Autodesk Inventor part; units mm, degrees
ref_plane "YZ Plane" through (0, 0, 0) normal (1, 0, 0) x (0, 1, 0)
ref_plane "XZ Plane" through (0, 0, 0) normal (0, 1, 0) x (-1, 0, 0)
ref_plane "XY Plane" through (0, 0, 0) normal (0, 0, 1) x (1, 0, 0)
sketch "Sketch1" plane through (0, 0, 0) normal (0, 1, 0) x (-1, 0, 0)
  circle A0 centre (0, 0) radius 69.85
  dimension "d0" = 139.7
extrude "Extrusion1" add sketch "Sketch1" along normal blind 29.21
sketch "Sketch3" plane through (0, 29.21, 0) normal (0, 1, 0) x (1, 0, 0)
  circle A0 centre (0, 0) radius 67.31
  dimension "d5" = 134.62
extrude "Extrusion2" cut sketch "Sketch3" against normal blind 26.67
sketch "Sketch6" plane through (0, 0, 0) normal (1, 0, 0) x (0, 1, 0)
  line L0 (29.21, 67.31) -> (2.54, 67.31)
  line L1 (29.21, 67.31) -> (27.686, 67.31)
  line L2 (27.686, 67.31) -> (27.686, 65.024)
  line L3 (27.686, 65.024) -> (29.21, 65.024)
  line L4 (29.21, 65.024) -> (29.21, 67.31)
  line L5 (-5.842, 0) -> (35.052, 0)
  line L6 (29.21, -69.85) -> (29.21, 69.85)
  point P0 (0, 0)
  dimension "d21" = 1.524
  dimension "d22" = 2.286
  dimension "d36" = 0
revolve "Revolution1" add sketch "Sketch6" angle 30 about axis through (0, -10, 0) along (0, 1, 0)
fillet "Fillet2" radius 0.762 2 edges at (16.8294, 27.686, 62.8084) (16.8294, 29.21, 62.8084)
fillet "Fillet3" radius 0.762 3 edges at (32.6235, 27.909, 56.5056) (33.2739, 29.21, 57.632) (33.2739, 27.686, 57.632)
pattern_circular "Circular Pattern1" count 3 over 360 about axis through (0, 0, 0) along (0, 1, 0) of "Revolution1", "Fillet2", "Fillet3"
sketch "Sketch9" plane through (0, 0, 0) normal (1, 0, 0) x (0, 1, 0)
  circle A0 centre (6.8717, 0) radius 3.175 construction
  line L0 (6.8717, 0) -> (6.8717, -12.7) construction
  line L1 (6.8717, 0) -> (6.8717, 12.7) construction
  line L2 (6.8717, -12.7) -> (6.8717, -12.7)
  line L3 (3.6967, -9.525) -> (3.6967, 9.525)
  line L4 (6.8717, 12.7) -> (6.8717, 12.7)
  line L5 (10.0467, 9.525) -> (10.0467, -9.525)
  arc A1 (6.8717, -12.7) -> (10.0467, -9.525) centre (6.8717, -9.525) ccw
  arc A2 (3.6967, -9.525) -> (6.8717, -12.7) centre (6.8717, -9.525) ccw
  arc A3 (6.8717, 12.7) -> (3.6967, 9.525) centre (6.8717, 9.525) ccw
  arc A4 (10.0467, 9.525) -> (6.8717, 12.7) centre (6.8717, 9.525) ccw
  point P0 (0, 0)
  dimension "d37" = 6.35
  dimension "d48" = 12.7
  dimension "d49" = 12.7
  dimension "d50" = 3.175
extrude "Extrusion9" cut sketch "Sketch9" along normal through all
sketch "Sketch20" plane through (0, 2.54, 0) normal (0, 1, 0) x (1, 0, 0)
  circle A0 centre (0, 0) radius 3.4925
  circle A1 centre (13.4366, 0) radius 24.638
  line L0 (38.0746, 0) -> (30.4546, 0) construction
  line L1 (30.4546, 0) -> (30.4546, -17.8162)
  line L2 (30.4546, 0) -> (30.4546, 17.8162)
  dimension "d70" = 6.985
  dimension "d71" = 49.276
  dimension "d72" = 13.4366
  dimension "d73" = 7.62
extrude "Extrusion13" add sketch "Sketch20" along normal blind 4.445 contours A0 | L2 L1 A1 picked at (19.7197, -7.6808)
properties part number "bottom_basket_2"
Build history of the part. All positions in model axes, mm. A direction names the side the tool comes from. Round coordinates to 2 decimals unless told otherwise and drop trailing zeros. Order: outer loops, then holes, each group sorted by start corner. A loop starts at its lowest first (then second) coordinate and runs counter-clockwise, first axis right, second up. Notation, with made-up numbers: M 55,14 L 96,14 A18 cw 96,22 Z; hole C 67.5,-0.75 d6. An arc over 180 degrees is marked long. Use CSV: the item, a comma, the result in double quotes. Start each with the question number.
(1) Drill centre lines: probe 1 along Z at (x, y) = (5.5, 5); probe 2 along Z at (x, y) = (0, 9.5); probe 3 along Z at (x, y) = (-42, 7). Where is each one in solid material? Low to high.
(2) Cut at B-B on y = 15.25. List the corners of the cut face in (x, z), then the cut area to 3 significant figures.
(3) Cut at C-C on z = 48. List the corners of the cut face in (x, y).
(4) Flat gauge pins, fed straight in: P1, Ø12.5, axis at x = 51, z = -41, coming from the -Y side; P2, Ø8, axis at y = 14, z = 11.5, coming from the -X side; P3, Ø6, axis at x = 39.5, y = 5.5, coming from the +Z side; P4, Ø8, axis at x = 25.5, z = 42, coming from the +Y side. Where does each tip first touch, or does it go through?
(5) Tool access for faces 4 (the face through (-14.59, 16.06, 65.71)), 5 (the face through (9, 6.985, 0)), 6 (the face through (67.6, 6.8, 12.7)), 7 (the face through (62.4, 29.21, 26.2)): list every direction of +Z, -Z, +X, -X, +Y, -Y with a clear straight run to the whole face (end or side of a thin tool).
(6) Cut at A-A on x = -20. List the corners of the cut face in (y, z).
(7) Mould opens along Z. For faces 1 (the face through (-66.624, 14.401, -20.981)), 2 (the face through (1, 0, 1)), 3 (the face through (68, 3.697, 0)) say: +Z half, -Z half, draft (parallel to the pull), parting line (faces both ways), or undercut.
Findings:
1,probe 1,"z = -69.63 to -67.08, -23.32 to 23.32, 67.08 to 69.63"
1,probe 2,"z = -69.85 to -67.31, 67.31 to 69.85"
1,probe 3,"z = -55.81 to -52.6, 52.6 to 55.81"
2,outline,"C 0,0 d139.7; hole C 0,0 d134.62"
2,area,"1,090 mm^2"
3,outline,"M -50.74,0 L 50.74,0 L 50.74,29.21 L 47.19,29.21 L 47.19,2.54 L -47.19,2.54 L -47.19,29.21 L -50.74,29.21 Z"
4,P1,"stops at y = 0"
4,P2,"stops at x = -69.45"
4,P3,"stops at z = 59.55"
4,P4,"stops at y = 2.54"
5,face 4,"none"
5,face 5,"+Y"
5,face 6,"+X"
5,face 7,"+Z, -Z, +X, -X, +Y"
6,outline,"M 0,-66.93 L 29.21,-66.93 L 29.21,-64.27 L 2.54,-64.27 L 2.54,64.27 L 29.21,64.27 L 29.21,66.93 L 0,66.93 Z"
7,face 1,"parting line"
7,face 2,"draft"
7,face 3,"undercut"
